```python
from build123d import *

# Parameters (mm, degrees)
F1_DEPTH = 3.2


with BuildPart() as f1:
    # F0 (on Top) → F1 (new body)
    with BuildSketch(Plane.XY):
        Polygon((-40, 28.15), (-60, 28.15), (-60, 18.15), (-56.8, 18.15), (-56.8, 8.15), (-60, 8.15), (-60, -1.85), (-56.8, -1.85), (-56.8, -11.85), (-60, -11.85), (-60, -21.85), (-40, -21.85), (-40, -18.65), (-20, -18.65), (-20, -21.85), (0, -21.85), (0, -18.65), (20, -18.65), (20, -21.85), (40, -21.85), (40, -18.65), (60, -18.65), (60, -21.85), (80, -21.85), (80, -18.65), (100, -18.65), (100, -21.85), (120, -21.85), (120, -18.65), (140, -18.65), (140, -5.65), (136.8, -5.65), (136.8, 11.95), (140, 11.95), (140, 24.95), (120, 24.95), (120, 28.15), (100, 28.15), (100, 24.95), (80, 24.95), (80, 28.15), (60, 28.15), (60, 24.95), (40, 24.95), (40, 28.15), (20, 28.15), (20, 24.95), (0, 24.95), (0, 28.15), (-20, 28.15), (-20, 24.95), (-40, 24.95), align=None)
        with BuildLine():
            ThreePointArc((-2.35, -10.65), (-4.9106601718, -11.7106601718), (-3.85, -9.15))
            ThreePointArc((-3.85, -9.15), (-2.7893398282, -9.5893398282), (-2.35, -10.65))
        make_face(mode=Mode.SUBTRACT)
        with BuildLine():
            ThreePointArc((19.9928815383, -10.6499136698), (17.4322213665, -11.7105738416), (18.4928815383, -9.1499136698))
            ThreePointArc((18.4928815383, -9.1499136698), (19.55354171, -9.589253498), (19.9928815383, -10.6499136698))
        make_face(mode=Mode.SUBTRACT)
        with BuildLine():
            ThreePointArc((-3.85, 8.15), (1.9129202667, 5.7629202667), (4.3, 0))
            ThreePointArc((4.3, 0), (1.9129202667, -5.7629202667), (-3.85, -8.15))
            ThreePointArc((-3.85, -8.15), (-12, 0), (-3.85, 8.15))
        make_face(mode=Mode.SUBTRACT)
        with BuildLine():
            ThreePointArc((18.4928815383, 8.1498871878), (24.2280612898, 5.7477393584), (26.6, 0))
            ThreePointArc((26.6, 0), (24.2280612898, -5.7477393584), (18.4928815383, -8.1498871878))
            ThreePointArc((18.4928815383, -8.1498871878), (10.3, 0), (18.4928815383, 8.1498871878))
        make_face(mode=Mode.SUBTRACT)
        with BuildLine():
            ThreePointArc((42.6330092816, -10.6431106304), (40.0723491098, -11.7037708021), (41.1330092816, -9.1431106304))
            ThreePointArc((41.1330092816, -9.1431106304), (42.1936694534, -9.5824504586), (42.6330092816, -10.6431106304))
        make_face(mode=Mode.SUBTRACT)
        with BuildLine():
            ThreePointArc((64.55, -10.65), (61.9893398282, -11.7106601718), (63.05, -9.15))
            ThreePointArc((63.05, -9.15), (64.1106601718, -9.5893398282), (64.55, -10.65))
        make_face(mode=Mode.SUBTRACT)
        with BuildLine():
            ThreePointArc((86.8551553416, -10.6499987522), (84.2944951698, -11.710658924), (85.3551553416, -9.1499987522))
            ThreePointArc((85.3551553416, -9.1499987522), (86.4158155134, -9.5893385804), (86.8551553416, -10.6499987522))
        make_face(mode=Mode.SUBTRACT)
        with BuildLine():
            ThreePointArc((41.1330092816, 8.1409952641), (46.6467798689, 5.6258765697), (48.9, 0))
            ThreePointArc((48.9, 0), (46.6467798689, -5.6258765697), (41.1330092816, -8.1409952641))
            ThreePointArc((41.1330092816, -8.1409952641), (32.6, 0), (41.1330092816, 8.1409952641))
        make_face(mode=Mode.SUBTRACT)
        with BuildLine():
            ThreePointArc((63.05, 8.15), (68.8129202667, 5.7629202667), (71.2, 0))
            ThreePointArc((71.2, 0), (68.8129202667, -5.7629202667), (63.05, -8.15))
            ThreePointArc((63.05, -8.15), (54.9, 0), (63.05, 8.15))
        make_face(mode=Mode.SUBTRACT)
        with BuildLine():
            ThreePointArc((85.3551553416, 8.1499983695), (91.114742667, 5.7610972898), (93.5, 0))
            ThreePointArc((93.5, 0), (91.114742667, -5.7610972898), (85.3551553416, -8.1499983695))
            ThreePointArc((85.3551553416, -8.1499983695), (77.2, 0), (85.3551553416, 8.1499983695))
        make_face(mode=Mode.SUBTRACT)
        with BuildLine():
            ThreePointArc((-2.35, 10.65), (-2.7893398282, 9.5893398282), (-3.85, 9.15))
            ThreePointArc((-3.85, 9.15), (-4.9106601718, 11.7106601718), (-2.35, 10.65))
        make_face(mode=Mode.SUBTRACT)
        with BuildLine():
            ThreePointArc((19.9928815383, 10.6499136698), (19.55354171, 9.589253498), (18.4928815383, 9.1499136698))
            ThreePointArc((18.4928815383, 9.1499136698), (17.4322213665, 11.7105738416), (19.9928815383, 10.6499136698))
        make_face(mode=Mode.SUBTRACT)
        with BuildLine():
            ThreePointArc((42.6330092816, 10.6431106304), (42.1936694534, 9.5824504586), (41.1330092816, 9.1431106304))
            ThreePointArc((41.1330092816, 9.1431106304), (40.0723491098, 11.7037708021), (42.6330092816, 10.6431106304))
        make_face(mode=Mode.SUBTRACT)
        with BuildLine():
            ThreePointArc((64.55, 10.65), (64.1106601718, 9.5893398282), (63.05, 9.15))
            ThreePointArc((63.05, 9.15), (61.9893398282, 11.7106601718), (64.55, 10.65))
        make_face(mode=Mode.SUBTRACT)
        with BuildLine():
            ThreePointArc((86.8551553416, 10.6499987522), (86.4158155134, 9.5893385804), (85.3551553416, 9.1499987522))
            ThreePointArc((85.3551553416, 9.1499987522), (84.2944951698, 11.710658924), (86.8551553416, 10.6499987522))
        make_face(mode=Mode.SUBTRACT)
    extrude(amount=F1_DEPTH)


solid = f1.part
```
Geometry: final body of the model. Coordinates: model frame, mm. A direction names the side the tool comes from. Round coordinates to 2 decimals unless told otherwise and drop trailing zeros. Order: outer loops, then holes, each group sorted by start corner. A loop starts at its lowest first (then second) coordinate and runs counter-clockwise, first axis right, second up. Notation, with made-up numbers: (85.5, 60.5) -> (130.5, 60.5) arc R25 ccw to (130.5, 85.5) -> close; hole circle Ø6 at (-13, 85.25). An arc over 180 degrees is marked (long way). Write each question's results on one line, items separated by ' | '.
Q1. Section query A-A (z = 1.65). Count the separate pieces of the cut face and the enclosed holes in it, and give its area (3 significant figures).
Response values:
separate pieces: 1 | enclosed holes: 15 | area: 8,130 mm²
Q2. Access query for faces 1 (the face through (120, -20, 2)), 2 (the face through (100, -20, 2)), 3 (the face through (-58, 18.15, 2)), 4 (the face through (90, 24.95, 2)), 5 (the face through (136.8, 3, 2)). Directions: +Z, -Z, +X, -X, +Y, -Y. A direction counts if a zero-diameter tool reaches every point of the face in a straight line with its end or side. Return the directions, or none.
Response values:
face 1: +Z, -Z, +X, -Y | face 2: +Z, -Z, -Y | face 3: +Z, -Z, -X | face 4: +Z, -Z, +Y | face 5: +Z, -Z, +X
Q3. Section query C-C (x = -23). Output: boundary loops of the cut face in (y, z).
Response values:
outline: (-18.65, 0) -> (24.95, 0) -> (24.95, 3.2) -> (-18.65, 3.2) -> close
Q4. Pin query (flat end, axial travel): pin 1 Ø1 at (y, z) = (-20, 2) entering from +X; pin 2 Ø2.5 at (x, y) = (-3.85, 10.65) entering from +Z; pin 3 Ø1 at (x, z) = (139, 2) entering from +Y; pin 4 Ø1 at (y, z) = (15.5, 2.5) entering from -X. Return the tip coordinate at first contact, or that it passes through.
Response values:
pin 1: x = 120 | pin 2: through | pin 3: y = 24.95 | pin 4: x = -56.8
Q5. Section query B-B (x = 69.5). Output: boundary loops of the cut face in (y, z), and give its area (3 significant figures).
Response values:
outline: (-21.85, 0) -> (-4.98, 0) -> (-4.98, 3.2) -> (-21.85, 3.2) -> close; (4.98, 0) -> (28.15, 0) -> (28.15, 3.2) -> (4.98, 3.2) -> close | area: 128 mm²
Q6. Pull-direction query (X, two-part tool) for faces 6 (the face through (-58, -1.85, 2)), 7 (the face through (50, 24.95, 2)), 8 (the face through (120, 27, 2)); classes: released by +X, released by -X, zero draft, split by the parting line, or undercut.
Response values:
face 6: zero draft | face 7: undercut | face 8: released by +X
Q7. Ray query, line 1 along Y through (x, z) = (63.05, 1.9); line 2 along X through (y, z) = (10.65, 0.95); line 3 along X through (y, z) = (10.5, 2.7). Return the intervals inside material, ascending.
Response values:
line 1: -21.85 to -12.15, -9.15 to -8.15, 8.15 to 9.15, 12.15 to 28.15 | line 2: -56.8 to -5.35, -2.35 to 16.99, 19.99 to 39.63, 42.63 to 61.55, 64.55 to 83.86, 86.86 to 136.8 | line 3: -56.8 to -5.34, -2.36 to 17, 19.99 to 39.64, 42.63 to 61.56, 64.54 to 83.86, 86.85 to 136.8
